For this review, take the finished solid that the model builds, in its own axes (mm). A direction names the side the tool comes from. Coordinates: 2 decimals unless noted, no trailing zeros. Write each loop counter-clockwise with the first axis right and the second up, starting at its lowest first coordinate (ties: lowest second). Pieces come first, ordered by that corner, then holes. Notation, with made-up numbers: M 52,49.5 L 98,49.5 A19 cw 98,75.5 Z; hole C -2,35 d3. An arc over 180 degrees is marked long. One line per question, with ' | ' between items.
from build123d import *

# Parameters (mm, degrees)
SKETCH1_R              = 27.5
BOTTOMLIP_DEPTH        = 7
SKETCH2_R              = 17.45
SKETCH2_R_2            = 11
UPPERRING_DEPTH        = 7
MIDDLEHOLE_START       = -7
SKETCH4_R              = 11
MIDDLEHOLE_DEPTH       = 7
SKETCH5_R              = 2
STATORHOLES_DEPTH      = 7
SKETCH6_R              = 13.5
INNERBEARINGHOLE_DEPTH = 6.5
SKETCH7_R              = 2.25
MOUNTINGHOLES_DEPTH    = 6
SKETCH8_R              = 3.5
CUT_EXTRUDE1_DEPTH     = 4


with BuildPart() as part:
    # Sketch1 → BottomLip (new body)
    with BuildSketch(Plane.XY):
        Circle(SKETCH1_R)
    extrude(amount=BOTTOMLIP_DEPTH)

    # Sketch2 → UpperRing (add)
    with BuildSketch(Plane.XY.offset(7)):
        Circle(SKETCH2_R)
        Circle(SKETCH2_R_2, mode=Mode.SUBTRACT)
    extrude(amount=UPPERRING_DEPTH)

    # Sketch4 → MiddleHole (cut)
    with BuildSketch(Plane.XY.offset(7).offset(MIDDLEHOLE_START)):
        Circle(SKETCH4_R)
    extrude(amount=MIDDLEHOLE_DEPTH, mode=Mode.SUBTRACT)

    # Sketch5 → StatorHoles (cut)
    with BuildSketch(Plane.XY.offset(7)):
        with Locations((23, 0)):
            Circle(SKETCH5_R)
        with Locations((7.107390871, -21.874299875)):
            Circle(SKETCH5_R)
        with Locations((-18.607390871, -13.519060803)):
            Circle(SKETCH5_R)
        with Locations((-18.607390871, 13.519060803)):
            Circle(SKETCH5_R)
        with Locations((7.107390871, 21.874299875)):
            Circle(SKETCH5_R)
    extrude(amount=-STATORHOLES_DEPTH, mode=Mode.SUBTRACT)

    # Sketch6 → InnerBearingHole (cut)
    with BuildSketch(Plane(origin=(0, 0, 0), x_dir=(-1, 0, 0), z_dir=(0, 0, -1))):
        Circle(SKETCH6_R)
    extrude(amount=-INNERBEARINGHOLE_DEPTH, mode=Mode.SUBTRACT)

    # Sketch7 → MountingHoles (cut)
    with BuildSketch(Plane.XY.offset(14)):
        with Locations((14.225, 0)):
            Circle(SKETCH7_R)
        with Locations((0, -14.5)):
            Circle(SKETCH7_R)
        with Locations((-14.5, -0.275)):
            Circle(SKETCH7_R)
        with Locations((-0.275, 14.225)):
            Circle(SKETCH7_R)
    extrude(amount=-MOUNTINGHOLES_DEPTH, mode=Mode.SUBTRACT)

    # Sketch8 → Cut-Extrude1 (cut)
    with BuildSketch(Plane.XY.offset(7)):
        with Locations((23, 0)):
            Circle(SKETCH8_R)
        with Locations((7.107390871, -21.874299875)):
            Circle(SKETCH8_R)
        with Locations((-18.607390871, -13.519060803)):
            Circle(SKETCH8_R)
        with Locations((-18.607390871, 13.519060803)):
            Circle(SKETCH8_R)
        with Locations((7.107390871, 21.874299875)):
            Circle(SKETCH8_R)
    extrude(amount=-CUT_EXTRUDE1_DEPTH, mode=Mode.SUBTRACT)


solid = part.part
1. For line 1 along X through (y, z) = (-12.5, 2); line 2 along Z through (x, y) = (14, -15.5); line 3 along X through (y, z) = (-11.5, 6.25), list the stretches that pass through material, from the lowest coordinate up.
Computed values:
line 1: x = -24.49 to -20.33, -16.89 to -5.1, 5.1 to 24.49 | line 2: z = 0 to 7 | line 3: x = -24.98 to -21.47, -15.75 to -7.07, 7.07 to 24.98
2. Clearance check with flat-ended pins moving along their axes: P1, Ø3, axis at x = -1.5, z = 5, coming from the +Y side; P2, Ø8, axis at x = 21.5, z = 1.5, coming from the -Y side; P3, Ø2, axis at x = 18, z = 2, coming from the +Y side. State where each tip first meets the part, or that it passes through.
Computed values:
P1: stops at y = 27.5 | P2: stops at y = -21.21 | P3: stops at y = 21.62
3. Machinability: for faces 1 (the cylindrical face through (21, 0, 2)), 2 (the flat face through (-15, 0, 8)), 3 (the flat face through (5, -10, 6.5)), which of the approach directions +Z, -Z, +X, -X, +Y, -Y give a long, thin tool a straight path to every point of the face, cutting with its end or side? Answer none if there is none.
Computed values:
face 1: +Z, -Z | face 2: +Z | face 3: -Z
4. Take a section at D-D on x = -10. State the section outline as (y, z) points, plus the area to 3 significant figures.
Computed values:
outline: M -25.62,0 L -9.07,0 L -9.07,6.5 L -4.58,6.5 L -4.58,14 L -14.3,14 L -14.3,7 L -25.62,7 Z; M 4.58,6.5 L 9.07,6.5 L 9.07,0 L 25.62,0 L 25.62,7 L 14.3,7 L 14.3,14 L 4.58,14 Z | area: 372 mm2
5. Take a section at B-B on y = -9. State the section outline as (x, z) points.
Computed values:
outline: M -25.99,0 L -10.06,0 L -10.06,6.5 L -6.32,6.5 L -6.32,14 L -14.95,14 L -14.95,7 L -25.99,7 Z; M 6.32,6.5 L 10.06,6.5 L 10.06,0 L 25.99,0 L 25.99,7 L 14.95,7 L 14.95,14 L 6.32,14 Z
6. Take a section at C-C on z = 5. State the section outline as (x, y) points, plus the area to 3 significant figures.
Computed values:
outline: C 0,0 d55; hole C -18.61,-13.52 d7; hole C -18.61,13.52 d7; hole C 0,0 d27; hole C 7.11,-21.87 d7; hole C 7.11,21.87 d7; hole C 23,0 d7 | area: 1,610 mm2
7. Draft analysis for pull direction X (two halves, no side actions). For faces 4 (the cylindrical face through (-5.961, -26.846, 3.451)), 5 (the flat face through (6, 13, 0)), 6 (the cylindrical face through (2.93, -13.18, 3.2)), state which applies: pulls with the +X half, pulls with the -X half, needs draft (parallel to the pull), parting line crosses it, or undercut.
Computed values:
face 4: parting line crosses it | face 5: needs draft | face 6: undercut
8. Take a section at A-A on x = 6. Give the number of separate pieces and of enclosed holes in the cut face, plus the area to 3 significant figures.
Computed values:
separate pieces: 4 | enclosed holes: 0 | area: 237 mm2
